Job drawing, mm, ordinate dimensions from the low corner. One solid piece. A direction names the side the tool comes from. Give positions to 0.01 mm unless a question says otherwise; leave off trailing zeros. Write each loop counter-clockwise with the first axis right and the second up, starting at its lowest first coordinate (ties: lowest second). Pieces come first, ordered by that corner, then holes. Notation, with made-up numbers: (56, -15.75) -> (65, -15.75) arc R12 cw to (65, 0.25) -> close; hole circle Ø11 at (-38, -13). An arc over 180 degrees is marked (long way). One line per question, with ' | ' between items. Start each with the question number.
(1) Pin check, flat tips, straight feed: P1, Ø5, axis at x = 10, z = 3.5, coming from the -Y side; P2, Ø2.5, axis at y = 24.5, z = 7, coming from the +X side; P3, Ø1.5, axis at y = 24.5, z = 3, coming from the +X side. Stop position of each tip, or through.
(2) Band-saw the part on D-D, the plane x = 67.5. Give the cut face in (y, z), and give its area (3 significant figures).
(3) Band-saw the part on B-B, the plane y = 12. Give the cut face in (x, z).
(4) Tool access for the marked faces 4, 5, 6, 7 and 8: list every direction of +Z, -Z, +X, -X, +Y, -Y with a clear straight run to the whole face (end or side of a thin tool).
(5) Band-saw the part on C-C, the plane z = 2.75. Give the cut face in (x, y).
(6) Band-saw the part on A-A, the plane z = 8.75. Give the cut face in (x, y).
(7) Pull direction X, two halves, no side cores. Call the marked faces 1, 2 and 3: released by +X, released by -X, zero draft, split by the parting line, or undercut.
(8) Drill centre lines: probe 1 along X at (y, z) = (28, 5.5); probe 2 along X at (y, z) = (27, 4). Where is each one in solid material? Low to high. Write a range as from..to.
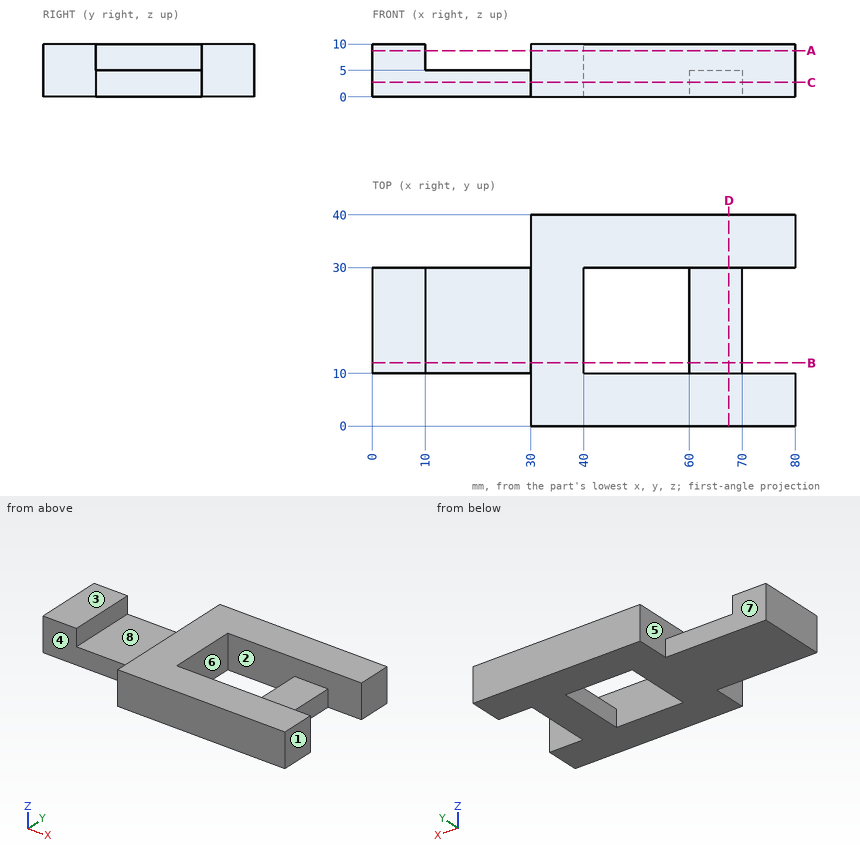
Results:
1) P1: stops at y = 10 | P2: stops at x = 40 | P3: stops at x = 70
2) outline: (0, 0) -> (40, 0) -> (40, 10) -> (30, 10) -> (30, 5) -> (10, 5) -> (10, 10) -> (0, 10) -> close | area: 300 mm²
3) outline: (0, 0) -> (40, 0) -> (40, 10) -> (30, 10) -> (30, 5) -> (10, 5) -> (10, 10) -> (0, 10) -> close; (60, 0) -> (70, 0) -> (70, 5) -> (60, 5) -> close
4) face 4: +Z, -Z, -X, -Y | face 5: +Z | face 6: +Z, -Z | face 7: +Z, -Z, -X, +Y | face 8: +Z, +Y, -Y
5) outline: (0, 10) -> (30, 10) -> (30, 0) -> (80, 0) -> (80, 10) -> (70, 10) -> (70, 30) -> (80, 30) -> (80, 40) -> (30, 40) -> (30, 30) -> (0, 30) -> close; hole (40, 10) -> (60, 10) -> (60, 30) -> (40, 30) -> close
6) outline: (0, 10) -> (10, 10) -> (10, 30) -> (0, 30) -> close; (30, 0) -> (80, 0) -> (80, 10) -> (40, 10) -> (40, 30) -> (80, 30) -> (80, 40) -> (30, 40) -> close
7) face 1: released by +X | face 2: undercut | face 3: zero draft
8) probe 1: x = 0..10, 30..40 | probe 2: x = 0..40, 60..70
